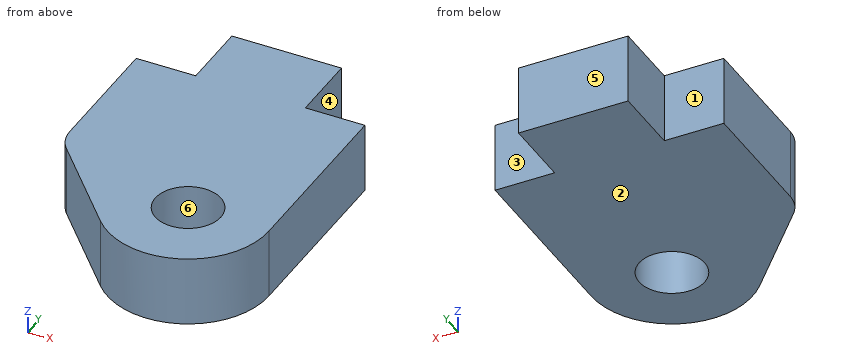
```python
from build123d import *

# Parameters (mm, degrees)
SKETCH1_R           = 1.4859
BOSS_EXTRUDE1_DEPTH = 3.175


with BuildPart() as part:
    # Sketch1 → Boss-Extrude1 (new body)
    with BuildSketch(Plane.XY):
        with BuildLine():
            Line((-4.744382059, -2.509411554), (-1.186842353, -6.436927856))
            ThreePointArc((-1.186842353, -6.436927856), (2.839838282, -7.394162612), (5.1816, -3.98145))
            Line((5.1816, -3.98145), (5.1816, 4.46405))
            Line((5.1816, 4.46405), (2.48285, 4.46405))
            Line((2.48285, 4.46405), (2.48285, 7.63905))
            Line((2.48285, 7.63905), (-2.48285, 7.63905))
            Line((-2.48285, 7.63905), (-2.48285, 4.46405))
            Line((-2.48285, 4.46405), (-5.1816, 4.46405))
            Line((-5.1816, 4.46405), (-5.1816, -1.375458239))
            ThreePointArc((-5.1816, -1.375458239), (-5.068509644, -1.983119668), (-4.744382059, -2.509411554))
        make_face()
        with Locations((1.524, -3.98145)):
            Circle(SKETCH1_R, mode=Mode.SUBTRACT)
    extrude(amount=BOSS_EXTRUDE1_DEPTH)


solid = part.part
```
Can you work these out from the model? Positions are in its coordinate system, mm. Face numbers are marked on the shaded views. A direction names the side the tool comes from. Give positions to 0.01 mm unless a question says otherwise; leave off trailing zeros. Loops run counter-clockwise (first coordinate to the right, second up) from the corner with the lowest first, then second, coordinate; pieces in that order, holes last. Notation, with made-up numbers: M 89.5,50 L 99.5,50 A19 ccw 99.5,84 Z; hole C 19,-39.5 d4. An arc over 180 degrees is marked long. Use one line per item in the form item = value. Start each with the question number.
(1) Please list where these lines run through material, in increasing order: line 1 (Y direction, x = 0.5, z = 2.7); line 2 (Y direction, x = -3, z = 2.45); line 3 (Y direction, x = -4, z = 2.4).
(2) I want a section at A-A, the plane z = 0.4. Write out the boundary of the cut face in (x, y).
(3) I want a section at D-D, the plane y = 5. Write out the boundary of the cut face in (x, z) (3 decimals), and give its area (3 significant figures).
(4) I'm going to push flat-ended pins straight in: P1, Ø1.6, axis at y = 6.5, z = 2, coming from the -X side; P2, Ø0.8, axis at x = 3.5, z = 2.5, coming from the +Y side. Where does each tip first touch, or does it pass through?
(5) I want a section at C-C, the plane x = 1.25. Write out the boundary of the cut face in (y, z) (3 decimals), and give its area (3 significant figures).
(6) I want a section at B-B, the plane y = -3. Write out the boundary of the cut face in (x, z) (3 decimals), and give its area (3 significant figures).
(7) On a 3-axis mill with a long thin cutter (end or side, diameter ignored), from which of +Z, -Z, +X, -X, +Y, -Y can I reach the whole of each face in a straight line? I mean the marked faces 1, 2 and 3. Say none if no direction works.
(8) Thinking about a two-plate mould opening in X: for the marked faces 4, 5 and 6, which applies, released by +X, released by -X, zero draft, split by the parting line, or undercut?
Worked out:
q1.line_1 = -7.49 to -5.06, -2.9 to 7.64
q1.line_2 = -4.44 to 4.46
q1.line_3 = -3.33 to 4.46
q2.outline = M -5.18,-1.38 A1.69 ccw -4.74,-2.51 L -1.19,-6.44 A3.66 ccw 5.18,-3.98 L 5.18,4.46 L 2.48,4.46 L 2.48,7.64 L -2.48,7.64 L -2.48,4.46 L -5.18,4.46 Z; hole C 1.52,-3.98 d2.97
q3.outline = M -2.483,0 L 2.483,0 L 2.483,3.175 L -2.483,3.175 Z
q3.area = 15.8 mm²
q4.P1 = -2.48
q4.P2 = 4.46
q5.outline = M -7.629,0 L -5.442,0 L -5.442,3.175 L -7.629,3.175 Z; M -2.521,0 L 7.639,0 L 7.639,3.175 L -2.521,3.175 Z
q5.area = 39.2 mm²
q6.outline = M -4.3,0 L 0.408,0 L 0.408,3.175 L -4.3,3.175 Z; M 2.64,0 L 5.182,0 L 5.182,3.175 L 2.64,3.175 Z
q6.area = 23.0 mm²
q7.face_1 = +Z, -Z, -X, +Y
q7.face_2 = -Z, +X, -X, +Y, -Y
q7.face_3 = +Z, -Z, +X, +Y
q8.face_4 = released by +X
q8.face_5 = zero draft
q8.face_6 = undercut
